Autodesk Inventor part; units mm, degrees
ref_plane "YZ Plane" through (0, 0, 0) normal (1, 0, 0) x (0, 1, 0)
ref_plane "XZ Plane" through (0, 0, 0) normal (0, 1, 0) x (-1, 0, 0)
ref_plane "XY Plane" through (0, 0, 0) normal (0, 0, 1) x (1, 0, 0)
sketch "Skizze1" plane through (0, 0, 0) normal (1, 0, 0) x (0, 1, 0)
  line L0 (0, 0) -> (198, 0)
  line L1 (198, 0) -> (198, 87)
  line L2 (198, 87) -> (0, 87)
  line L3 (0, 87) -> (0, 0)
  dimension "d0" = 198
  dimension "d1" = 87
extrude "Extrusion1" add sketch "Skizze1" along normal blind 10
sketch "Skizze2" plane through (10, 0, 0) normal (1, 0, 0) x (0, 0, -1)
  line L0 (-87, 0) -> (0, 0)
  line L1 (-80.5, 147.5) -> (-80.5, 50.5) construction
  line L2 (0, 0) -> (0, 198)
  dimension "d4" = 97
  dimension "d5" = 50.5
  dimension "d6" = 80.5
hole "Bohrung1" at (10, 147.5, 80.5) at (10, 50.5, 80.5) direction (-1, 0, 0) diameter 4.2 depth 10
sketch "Skizze3" plane through (10, 0, 0) normal (1, 0, 0) x (0, 0, -1)
  circle A0 centre (-80.5, 147.5) radius 2.1
  circle A1 centre (-80.5, 50.5) radius 2.1
  arc A2 (-87, 50.5) -> (-84.2395, 45.1834) centre (-80.5, 50.5) ccw
  arc A3 (-84.2395, 152.8166) -> (-87, 147.5) centre (-80.5, 147.5) ccw
  line L0 (0, 0) -> (0, 198)
  line L1 (0, 198) -> (-20, 198) construction
  line L2 (0, 0) -> (-20, 0) construction
  line L3 (-87, 0) -> (0, 0)
  line L4 (-20, 0) -> (-84.2395, 45.1834)
  line L5 (-20, 198) -> (-84.2395, 152.8166)
  line L6 (-87, 198) -> (-87, 0)
  line L7 (-20, 198) -> (-87, 198)
  line L8 (-87, 147.5) -> (-87, 198)
  line L9 (-87, 50.5) -> (-87, 0)
  line L10 (-87, 0) -> (-20, 0)
  dimension "d15" = 20
extrude "Extrusion2" cut sketch "Skizze3" against normal up to surface (10 mm away) contours L6 L7 L5 A3 | A2 L4 L3 L6
sketch "Skizze4" plane through (10, 0, 0) normal (1, 0, 0) x (0, 0, -1)
  line L0 (0, 0) -> (0, 198)
  line L1 (-20, 0) -> (0, 0)
  line L2 (0, 198) -> (-20, 198)
  line L3 (-87, 147.5) -> (-87, 50.5)
  line L4 (-87, 99) -> (0, 99)
  point P0 (-10, 10)
  point P1 (-10, 188)
  point P2 (-10, 99)
  dimension "d18" = 10
  dimension "d19" = 10
  dimension "d20" = 10
hole "Bohrung2" at (10, 10, 10) at (10, 188, 10) at (10, 99, 10) direction (-1, 0, 0) diameter 4.5 end through all counterbore diameter 8 counterbore depth 5
fillet "Rundung1" radius 5 4 edges at (5, 198, 20) (5, 0, 20) (5, 0, 0) (5, 198, 0)
properties part number "102.006.01_Anbindung_Aktor"
Part model, mm, in its own coordinate system. A direction names the side the tool comes from. Give positions to 0.01 mm unless a question says otherwise; leave off trailing zeros. Loops run counter-clockwise (first coordinate to the right, second up) from the corner with the lowest first, then second, coordinate; pieces in that order, holes last. Notation, with made-up numbers: M 33.25,63 L 42.25,63 A8 ccw 42.25,68 Z; hole C 52.5,28.5 d5. An arc over 180 degrees is marked long. Return JSON: item names as keys, results as strings.
1) Saw through at D-D, the plane z = 80.5. List the corners of the cut face in (x, y), then the cut area to 3 significant figures.
Calculated:
{"outline": "M 0,42.55 L 10,42.55 L 10,48.4 L 0,48.4 Z; M 0,52.6 L 10,52.6 L 10,145.4 L 0,145.4 Z; M 0,149.6 L 10,149.6 L 10,155.45 L 0,155.45 Z", "area": "1,040 mm2"}
2) Saw through at B-B, the plane y = 99. List the corners of the cut face in (x, z).
Calculated:
{"outline": "M 0,0 L 10,0 L 10,6 L 5,6 L 5,7.75 L 0,7.75 Z; M 0,12.25 L 5,12.25 L 5,14 L 10,14 L 10,87 L 0,87 Z"}
3) 3-axis set-ups, long thin cutter, end or side, ignore diameter. For faces 1 (the face through (5, 190, 8)), 2 (the face through (4.93, 146.081, 82.048)): which of +Z, -Z, +X, -X, +Y, -Y reach the whole face in a straight line?
Calculated:
{"face 1": "+X", "face 2": "+X, -X"}
4) Saw through at C-C, the plane x = 7.25. List the corners of the cut face in (y, z).
Calculated:
{"outline": "M 0,5 A5 ccw 5,0 L 193,0 A5 ccw 198,5 L 198,18.42 A5 ccw 197.09,21.29 L 152.82,84.24 A6.5 ccw 147.5,87 L 50.5,87 A6.5 ccw 45.18,84.24 L 0.91,21.29 A5 ccw 0,18.42 Z; hole C 10,10 d8; hole C 50.5,80.5 d4.2; hole C 99,10 d8; hole C 147.5,80.5 d4.2; hole C 188,10 d8"}
5) Flat gauge pins, fed straight in: pin 1 Ø7 at (y, z) = (188, 10) entering from +X; pin 2 Ø5 at (x, z) = (1.5, 58) entering from +Y; pin 3 Ø1.5 at (x, z) = (6, 26) entering from +Y. Where does each tip first touch, or does it go through?
Calculated:
{"pin 1": "stops at x = 5", "pin 2": "stops at y = 173.03", "pin 3": "stops at y = 194.31"}
6) Drill centre lines: line 1 (Y direction, x = 8.25, z = 10); line 2 (Y direction, x = 4.05, z = 10); line 3 (Z direction, x = 2.25, y = 147.5). Where is each one in solid material? Low to high.
Calculated:
{"line 1": "y = 0 to 6, 14 to 95, 103 to 184, 192 to 198", "line 2": "y = 0 to 7.75, 12.25 to 96.75, 101.25 to 185.75, 190.25 to 198", "line 3": "z = 0 to 78.4, 82.6 to 87"}
7) Pull direction Z, two halves, no side cores. Call faces 3 (the face through (5, 196, 1)), 4 (the face through (5, 100, 87)), 5 (the face through (0, 98, 34)), 6 (the face through (5, 12, 8)): released by +Z, released by -Z, zero draft, split by the parting line, or undercut.
Calculated:
{"face 3": "released by -Z", "face 4": "released by +Z", "face 5": "zero draft", "face 6": "undercut"}
8) Saw through at A-A, the plane z = 10. List the corners of the cut face in (x, y).
Calculated:
{"outline": "M 0,0 L 10,0 L 10,6 L 5,6 L 5,7.75 L 0,7.75 Z; M 0,12.25 L 5,12.25 L 5,14 L 10,14 L 10,95 L 5,95 L 5,96.75 L 0,96.75 Z; M 0,101.25 L 5,101.25 L 5,103 L 10,103 L 10,184 L 5,184 L 5,185.75 L 0,185.75 Z; M 0,190.25 L 5,190.25 L 5,192 L 10,192 L 10,198 L 0,198 Z"}
